Can you work these out from the model? Positions are in its coordinate system, mm. A direction names the side the tool comes from. Coordinates: 2 decimals unless noted, no trailing zeros. Order: outer loops, then holes, each group sorted by start corner. A loop starts at its lowest first (then second) coordinate and runs counter-clockwise, first axis right, second up.
```python
from build123d import *

# Parameters (mm, degrees)
SKETCH1_R           = 19.05
BOSS_EXTRUDE1_DEPTH = 12.7
SKETCH2_R           = 9.525
BOSS_EXTRUDE2_DEPTH = 38.1
SKETCH3_R           = 6.985
CUT_EXTRUDE1_DEPTH  = 46.99
CUT_EXTRUDE2_DEPTH  = 19.05


with BuildPart() as part:
    # Sketch1 → Boss-Extrude1 (new body)
    with BuildSketch(Plane(origin=(0, 0, 0), x_dir=(1, 0, 0), z_dir=(0, 1, 0))):
        Circle(SKETCH1_R)
    extrude(amount=BOSS_EXTRUDE1_DEPTH)

    # Sketch2 → Boss-Extrude2 (add)
    with BuildSketch(Plane.XZ):
        Circle(SKETCH2_R)
    extrude(amount=BOSS_EXTRUDE2_DEPTH)

    # Sketch3 → Cut-Extrude1 (cut)
    with BuildSketch(Plane.XZ.offset(38.1)):
        Circle(SKETCH3_R)
    extrude(amount=-CUT_EXTRUDE1_DEPTH, mode=Mode.SUBTRACT)

    # Sketch5 → Cut-Extrude2 (cut)
    with BuildSketch(Plane.XZ.offset(-8.89)):
        with BuildLine():
            Line((0, 6.957071705), (19.05, 6.957071705))
            ThreePointArc((19.05, 6.957071705), (26.007071705, 0), (19.05, -6.957071705))
            Line((19.05, -6.957071705), (0, -6.957071705))
            ThreePointArc((0, -6.957071705), (-6.957071705, 0), (0, 6.957071705))
        make_face()
    extrude(amount=CUT_EXTRUDE2_DEPTH, mode=Mode.SUBTRACT)


solid = part.part
```
1. Imagine slicing it at B-B on x = 0. Please give me the cut outline in (y, z) (3 decimals), then the cut area to 3 significant figures.
Completed:
outline: (-38.1, -9.525) - (0, -9.525) - (0, -19.05) - (12.7, -19.05) - (12.7, 19.05) - (0, 19.05) - (0, 9.525) - (-38.1, 9.525) - (-38.1, 6.985) - (8.89, 6.985) - (8.89, -6.985) - (-38.1, -6.985) - close
area: 553 mm2
2. Thinking about a two-plate mould opening in Z: for faces 4 (the flat face through (-0.8, -38.1, 7.1)), 5 (the flat face through (7.4, -10.16, 0)), 6 (the cylindrical face through (-9.516, -18.783, 0.419)), which applies, pulls with the +Z half, pulls with the -Z half, needs draft (parallel to the pull), parting line crosses it, or undercut?
Completed:
face 4: needs draft
face 5: undercut
face 6: parting line crosses it
3. I'm going to push flat-ended pins straight in: pin 1 (6 mm diameter, centred on x = 8.5, y = -29, fed in from -Z); pin 2 (8 mm diameter, centred on y = -24.5, z = -10.5, fed in from +X); pin 3 (4 mm diameter, centred on y = -12.5, z = 3, fed in from -X). Where does each tip first touch, or does it pass through?
Completed:
pin 1: stops at z = -7.78
pin 2: stops at x = 6.96
pin 3: stops at x = -9.47
4. Imagine slicing it at D-D on x = 5. Please give me the cut outline in (y, z).
Completed:
outline: (-38.1, -8.11) - (0, -8.11) - (0, -18.38) - (12.7, -18.38) - (12.7, 18.38) - (0, 18.38) - (0, 8.11) - (-38.1, 8.11) - (-38.1, 4.88) - (-10.16, 4.88) - (-10.16, 6.96) - (8.89, 6.96) - (8.89, -6.96) - (-10.16, -6.96) - (-10.16, -4.88) - (-38.1, -4.88) - close
5. Imagine slicing it at C-C on y = -19.5. Please give me the cut outline in (x, z) (3 decimals), then the cut area to 3 significant figures.
Completed:
outline: circle Ø19.05 at (0, 0); hole circle Ø13.97 at (0, 0)
area: 132 mm2
6. Please list where these lines run through material, in increasing order: probe 1 along Z at (x, y) = (0, -6) (3 decimals); probe 2 along Y at (x, z) = (11, -15).
Completed:
probe 1: z = -9.525 to -6.985, 6.985 to 9.525
probe 2: y = 0 to 12.7
7. On a 3-axis mill with a long thin cutter (end or side, diameter ignored), from which of +Z, -Z, +X, -X, +Y, -Y can I reach the whole of each face in a straight line? I mean faces 1 (the cylindrical face through (-6.98, -20.16, 0.31)), 2 (the cylindrical face through (-15.12, 6.26, 11.59)), 3 (the flat face through (7, 2, -6.957)). Say none if no direction works.
Completed:
face 1: -Y
face 2: +Y, -Y
face 3: +X
8. Imagine slicing it at A-A on z = 0. Please give me the cut outline in (x, y) (3 decimals), then the cut area to 3 significant figures.
Completed:
outline: (-19.05, 0) - (-9.525, 0) - (-9.525, -38.1) - (-6.985, -38.1) - (-6.985, 8.89) - (19.05, 8.89) - (19.05, 12.7) - (-19.05, 12.7) - close; (6.985, -38.1) - (9.525, -38.1) - (9.525, -10.16) - (6.985, -10.16) - close
area: 420 mm2
